Drawing for the job (mm, zero at the part's lowest x, y, z). A direction names the side the tool comes from. Give positions to 0.01 mm unless a question says otherwise; leave off trailing zeros. Loops run counter-clockwise (first coordinate to the right, second up) from the corner with the lowest first, then second, coordinate; pieces in that order, holes last. Notation, with made-up numbers: (16, 58) - (30, 58) arc R23 cw to (30, 97) - close; hole circle Ø4 at (85, -36). An arc over 180 degrees is marked (long way). Return JSON: item names as keys, results as strings. Group by question number.
1) 3-axis set-ups, long thin cutter, end or side, ignore diameter. For the marked faces 1 and 2: which of +Z, -Z, +X, -X, +Y, -Y reach the whole face in a straight line?
2) Drop flat-ended pins along their axis: pin 1 (4 mm diameter, centred on x = 64.5, z = 8, fed in from +Y); pin 2 (0.6 mm diameter, centred on x = 45.5, z = 16, fed in from -Y) (1 decimal); pin 3 (4 mm diameter, centred on x = 60.5, y = 11, fed in from +Z). Give the stop position or say it passes through.
3) Slice it at B-B (z = 10). List the corners of the cut face in (x, y).
4) Drill centre lines: probe 1 along X at (y, z) = (5, 18.5); probe 2 along Y at (x, z) = (113, 14.75); probe 3 along Y at (x, z) = (37, 14) (1 decimal). Where is each one in solid material? Low to high. Write a range as from..to.
5) Slice it at C-C (x = 109). List the corners of the cut face in (y, z).
6) Slice it at D-D (x = 40.5). List the corners of the cut face in (y, z), and give its area (3 significant figures).
7) Slice it at A-A (y = 10). List the corners of the cut face in (x, z).
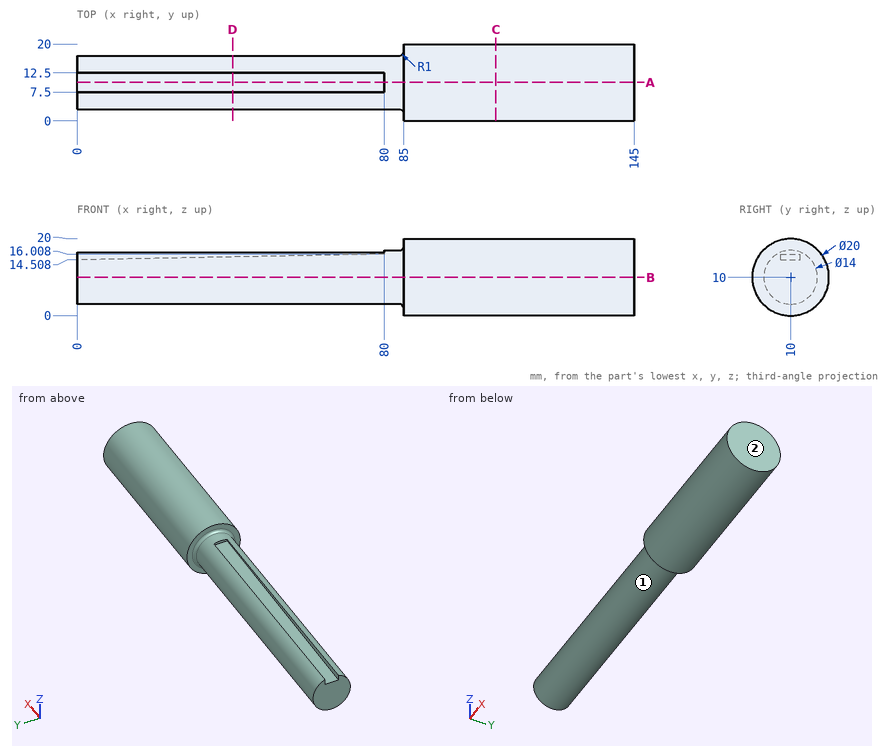
Results:
{
 "1": {"face 1": "-X", "face 2": "+Z, -Z, +X, +Y, -Y"},
 "2": {"pin 1": "y = 17", "pin 2": "y = 5.9", "pin 3": "z = 16.54"},
 "3": {"outline": "(0, 3) - (84, 3) arc R1 cw to (85, 2) - (85, 0) - (145, 0) - (145, 20) - (85, 20) - (85, 18) arc R1 cw to (84, 17) - (0, 17) - close"},
 "4": {"probe 1": "85..145", "probe 2": "1.2..18.8", "probe 3": "4.3..15.7"},
 "5": {"outline": "circle Ø20 at (10, 10)"},
 "6": {"outline": "(7.5, 15.27) - (7.5, 16.54) arc R7 ccw (long way) to (12.5, 16.54) - (12.5, 15.27) - close", "area": "146 mm2"},
 "7": {"outline": "(0, 3) - (84, 3) arc R1 cw to (85, 2) - (85, 0) - (145, 0) - (145, 20) - (85, 20) - (85, 18) arc R1 cw to (84, 17) - (80, 17) - (80, 16.01) - (0, 14.51) - close"}
}
